Work out the finished part from the listing and answer in its coordinate system (mm). Face numbers are marked on the shaded views. A direction names the side the tool comes from. Round coordinates to 2 decimals unless told otherwise and drop trailing zeros. Loops run counter-clockwise (first coordinate to the right, second up) from the corner with the lowest first, then second, coordinate; pieces in that order, holes last. Notation, with made-up numbers: (37.25, 50.25) -> (82.25, 50.25) arc R25 ccw to (82.25, 88.25) -> close; hole circle Ø7 at (-39.5, 77.25). An arc over 180 degrees is marked (long way). Use one line per item in the form item = value.
```python
from build123d import *

# Parameters (mm, degrees)
BOSS_EXTRUDE1_DEPTH     = 0.5
CIRPATTERN3_COUNT       = 20
CUT_EXTRUDE1_DEPTH      = 1
CUT_EXTRUDE1_DEPTH_BACK = 3.05


with BuildPart() as part:
    # Sketch1 → Revolve1 (revolve)
    with BuildSketch(Plane(origin=(0, 0, 0), x_dir=(0, 0, -1), z_dir=(1, 0, 0))):
        Polygon((-3.5, 0.525), (-3.5, -0.525), (-5, -0.525), (-5, -1.025), (0, -1.025), (0, -0.525), (0, 0.525), (0, 1.025), (-5, 1.025), (-5, 0.525), align=None)
    revolve(axis=Axis((0, 0, 0), (0, -1, 0)))

    # Sketch3 → Boss-Extrude1 (add)
    with BuildSketch(Plane.XZ.offset(1.025)):
        with BuildLine():
            ThreePointArc((-0.75, 4.943429983), (0, 5.193429983), (0.75, 4.943429983))
            ThreePointArc((0.75, 4.943429983), (0, 5), (-0.75, 4.943429983))
        make_face()
    boss_extrude1 = extrude(amount=-BOSS_EXTRUDE1_DEPTH)

    # CirPattern3: Boss-Extrude1 ×20 about axis
    cirpattern3_axis = Axis((0, 0, 0), (0, 1, 0))
    for i in range(1, CIRPATTERN3_COUNT):
        add(boss_extrude1.rotate(cirpattern3_axis, i * 360 / CIRPATTERN3_COUNT))

    # Sketch4 → Cut-Extrude1 (cut, two sides)
    with BuildSketch(Plane(origin=(0, 1.025, 0), x_dir=(1, 0, 0), z_dir=(0, 1, 0))) as cut_extrude1_sk:
        Polygon((1.299038106, 2.25), (-1.299038106, 2.25), (-2.598076211, 0), (-1.299038106, -2.25), (1.299038106, -2.25), (2.598076211, 0), align=None)
    extrude(amount=CUT_EXTRUDE1_DEPTH, mode=Mode.SUBTRACT)
    extrude(cut_extrude1_sk.sketch, amount=-CUT_EXTRUDE1_DEPTH_BACK, mode=Mode.SUBTRACT)


solid = part.part
```
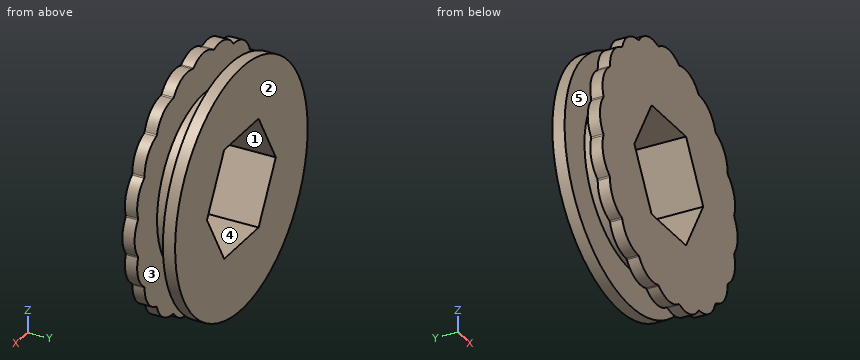
(1) Find section D-D, the plane x = -1.75. Write down the section's boundary in (y, z) (3 decimals).
Completed:
outline = (-1.025, -4.882) -> (-0.525, -4.882) -> (-0.525, -3.031) -> (0.525, -3.031) -> (0.525, -4.684) -> (1.025, -4.684) -> (1.025, -1.469) -> (-1.025, -1.469) -> close; (-1.025, 1.469) -> (1.025, 1.469) -> (1.025, 4.684) -> (0.525, 4.684) -> (0.525, 3.031) -> (-0.525, 3.031) -> (-0.525, 4.882) -> (-1.025, 4.882) -> close
(2) Find section C-C, the plane z = -4. Write down the section's boundary in (x, y) (3 decimals).
Completed:
outline = (-3.27, -1.025) -> (3.27, -1.025) -> (3.27, -0.525) -> (-3.27, -0.525) -> close; (-3, 0.525) -> (3, 0.525) -> (3, 1.025) -> (-3, 1.025) -> close
(3) Find section A-A, the plane x = 0. Write down the section's boundary in (y, z) (3 decimals).
Completed:
outline = (-1.025, -5.193) -> (-0.525, -5.193) -> (-0.525, -3.5) -> (0.525, -3.5) -> (0.525, -5) -> (1.025, -5) -> (1.025, -2.25) -> (-1.025, -2.25) -> close; (-1.025, 2.25) -> (1.025, 2.25) -> (1.025, 5) -> (0.525, 5) -> (0.525, 3.5) -> (-0.525, 3.5) -> (-0.525, 5.193) -> (-1.025, 5.193) -> close
(4) Given P1, Ø0.6, axis at x = 0, y = 0, coming from the -Z side; P2, Ø1, axis at x = 4, y = 0.5, coming from the -Z side; P3, Ø5, axis at x = -1.5, z = 0.5, coming from the -Y side (3 decimals), each flat-ended and moving along its own axis, determine where each tip first touches the part or whether it passes through.
Completed:
P1 = -3.5
P2 = -3.57
P3 = -1.025
(5) Find section B-B, the plane y = -0.2. Write down the section's boundary in (x, z), then the cut area to 3 significant figures.
Completed:
outline = circle Ø7 at (0, 0); hole (-2.6, 0) -> (-1.3, -2.25) -> (1.3, -2.25) -> (2.6, 0) -> (1.3, 2.25) -> (-1.3, 2.25) -> close
area = 20.9 mm2
(6) Consider L1, parallel to Y at x = 3.25, z = -2 (3 decimals); L2, parallel to Z at x = 2.5, y = 0.1; L3, parallel to Z at x = -1.75, y = -0.8. Determine where each line is inside the solid, lowest interval first.
Completed:
L1 = -1.025 to -0.525, 0.525 to 1.025
L2 = -2.45 to -0.17, 0.17 to 2.45
L3 = -4.88 to -1.47, 1.47 to 4.88
(7) For the marked faces 1, 2 and 3, determine the directions among +Z, -Z, +X, -X, +Y, -Y from which every point of the face is accessible in a straight line to the end or side of a thin tool.
Completed:
face_1 = +Y, -Y
face_2 = +Z, -Z, +X, -X, +Y
face_3 = none
(8) For a pull along X with two mould halves and no side action, classify the marked faces 4 and 5 as +X half, -X half, draft (parallel to the pull), parting line (faces both ways), or undercut.
Completed:
face_4 = undercut
face_5 = draft
